Model file for the job. Use its own axes, mm. Face numbers are marked on the shaded views. A direction names the side the tool comes from. Coordinates: 2 decimals unless noted, no trailing zeros. Write each loop counter-clockwise with the first axis right and the second up, starting at its lowest first coordinate (ties: lowest second). Pieces come first, ordered by that corner, then holes. Notation, with made-up numbers: (39, -9) - (48, -9) arc R20 cw to (48, 6) - close; hole circle Ø6 at (-27, 87.5). An arc over 180 degrees is marked (long way). Put each result on its own line as item: value. Start each with the question number.
1. Drill centre lines: L1, parallel to X at y = 6.75, z = 7.5; L2, parallel to X at y = 5.25, z = 1.5; L3, parallel to Y at x = -12, z = 2.75. Where is each one in solid material? Low to high. Write a range as from..to.
2. Saw through at D-D, the plane z = 6.5. Write the cut outline in (x, y).
3. Drop flat-ended pins along their axis: P1, Ø2, axis at y = -2.5, z = 5.5, coming from the -X side; P2, Ø4, axis at x = -14.5, z = 6, coming from the -Y side. Give the stop position or say it passes through.
4. Pull direction X, two halves, no side cores. Call the marked faces 3, 4 and 5: released by +X, released by -X, zero draft, split by the parting line, or undercut.
5. Saw through at A-A, the plane z = 4.5. Write the cut outline in (x, y), plus the area to 3 significant figures.
6. Saw through at C-C, the plane x = 6. Write the cut outline in (y, z), plus the area to 3 significant figures.
7. Saw through at B-B, the plane y = -7. Write the cut outline in (x, z), plus the area to 3 significant figures.
8. Which spindle directions (+Z, -Z, +X, -X, +Y, -Y) get a long thin tool onto all of the face, cutting with end or side? Do the marked faces 1 and 2. Say none if no direction does.
```python
from build123d import *

# Parameters (mm, degrees)
F0_W           = 40
F0_H           = 20
F1_DEPTH       = 10
F3_DEPTH       = 25
F5_D           = 3.3
F5_CSINK_D     = 6.72
F5_CSINK_ANGLE = 90
F6_T1_DEPTH    = 55


# Not quite as in the source:
# - a fillet or chamfer that OpenCascade refuses, or shapes differently, is made with other operations: its cross-section is extruded or revolved along the edge and cut away or added


with BuildPart() as f1:
    # F0 (on Top) → F1 (new body)
    with BuildSketch(Plane.XY):
        Rectangle(F0_W, F0_H)
    extrude(amount=F1_DEPTH)

    # F2 (on face) → F3 (cut)
    with BuildSketch(Plane.XY.offset(10)):
        Polygon((0, -8), (6.9282032303, -4), (6.9282032303, 4), (0, 8), (-6.9282032303, 4), (-6.9282032303, -4), align=None)
        with BuildLine():
            ThreePointArc((-10, -10), (-12.9289321881, -2.9289321881), (-20, 0))
            Line((-20, 0), (-20, -10))
            Line((-20, -10), (-10, -10))
        make_face()
        with BuildLine():
            Line((20, 10), (10, 10))
            ThreePointArc((10, 10), (12.9289321881, 2.9289321881), (20, 0))
            Line((20, 0), (20, 10))
        make_face()
    extrude(amount=-F3_DEPTH, mode=Mode.SUBTRACT)

    # F5 (through all)
    with Locations(Plane.XY.offset(10)):
        with Locations((-14.633436854, 7.316718427), (-9.266873708, 4.633436854)):
            CounterSinkHole(F5_D / 2, F5_CSINK_D / 2, counter_sink_angle=F5_CSINK_ANGLE)

    # F6: fillet of radius 5 on 1 edges, made by hand

    # F6_s2 → F6_t1 (cut)
    with BuildSketch(Plane.YZ.offset(-22.5)):
        with BuildLine():
            ThreePointArc((-10, 5), (-8.5355339059, 8.5355339059), (-5, 10))
            Line((-5, 10), (-10, 10))
            Line((-10, 10), (-10, 5))
        make_face()
    extrude(amount=F6_T1_DEPTH, mode=Mode.SUBTRACT)


solid = f1.part
```
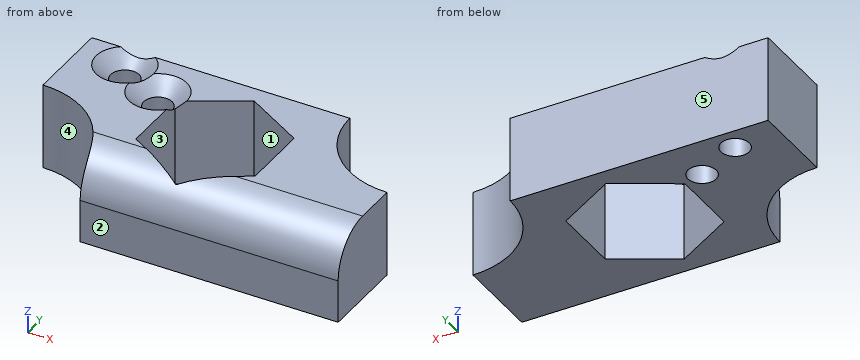
Final values:
1. L1: x = -20..-16.18, -13.08..-2.17, 2.17..10.54
1. L2: x = -20..-10.8, -7.74..-4.76, 4.76..11.2
1. L3: y = -4..10
2. outline: (-20, 0) arc R10 cw to (-10, -9.77) - (20, -9.77) - (20, 0) arc R10 cw to (10, 10) - (-20, 10) - close; hole circle Ø3.3 at (-14.63, 7.32); hole circle Ø3.3 at (-9.27, 4.63); hole (-6.93, -4) - (0, -8) - (6.93, -4) - (6.93, 4) - (0, 8) - (-6.93, 4) - close
3. P1: stops at x = -14.73
3. P2: stops at y = -3.39
4. face 3: undercut
4. face 4: released by -X
4. face 5: zero draft
5. outline: (-20, 0) arc R10 cw to (-10, -10) - (20, -10) - (20, 0) arc R10 cw to (10, 10) - (-20, 10) - close; hole circle Ø3.3 at (-14.63, 7.32); hole circle Ø3.3 at (-9.27, 4.63); hole (-6.93, -4) - (0, -8) - (6.93, -4) - (6.93, 4) - (0, 8) - (-6.93, 4) - close
5. area: 460 mm²
6. outline: (-10, 0) - (-4.54, 0) - (-4.54, 10) - (-5, 10) arc R5 ccw to (-10, 5) - close; (4.54, 0) - (10, 0) - (10, 10) - (4.54, 10) - close
6. area: 104 mm²
7. outline: (-10.46, 0) - (-1.73, 0) - (-1.73, 9.58) - (-10.46, 9.58) - close; (1.73, 0) - (20, 0) - (20, 9.58) - (1.73, 9.58) - close
7. area: 259 mm²
8. face 1: +Z, -Z
8. face 2: +Z, -Z, +X, -X, -Y
